```python
from build123d import *

# Parameters (mm, degrees)
SKETCH1_W                                  = 38
SKETCH1_H                                  = 38
BOSS_EXTRUDE1_DEPTH                        = 2
SKETCH2_R                                  = 2.25
BOSS_EXTRUDE2_DEPTH                        = 2
M3_TAPPED_HOLE1_D                          = 2.5
FILLET1_R                                  = 4
BOSS_EXTRUDE3_DEPTH                        = 1.5
SKETCH9_W                                  = 1.25
SKETCH9_H                                  = 1.5
SKETCH7_W                                  = 4.5
SKETCH7_H                                  = 2
BOSS_EXTRUDE4_DEPTH                        = 18
MIRROR1_AT_THE_SECOND_PLANE_COPY_1_SKETC_R = 2.25
MIRROR1_AT_THE_SECOND_PLANE_COPY_1_DEPTH   = 2
MIRROR1_AT_THE_SECOND_PLANE_COPY_2_D       = 2.5
MIRROR3_OUTLINE_W                          = 4.5
MIRROR3_OUTLINE_H                          = 2
MIRROR3_DEPTH                              = 19.5
MIRROR3_2_OUTLINE_R                        = 1.25
MIRROR3_2_DEPTH                            = 1.5


# Read off the part's stored shape, not the designer's step: Mirror3
with BuildPart() as part:
    # Sketch1 → Boss-Extrude1 (new body)
    with BuildSketch(Plane(origin=(0, 17.5, 0), x_dir=(1, 0, 0), z_dir=(0, 1, 0))):
        Rectangle(SKETCH1_W, SKETCH1_H)
    extrude(amount=BOSS_EXTRUDE1_DEPTH)

    # Sketch2 → Boss-Extrude2 (add)
    with BuildSketch(Plane(origin=(0, 19.5, 0), x_dir=(1, 0, 0), z_dir=(0, 1, 0))):
        with Locations(Location((15.25, 15.25, 0), (0, 0, 90))):
            Circle(SKETCH2_R)
    boss_extrude2 = extrude(amount=BOSS_EXTRUDE2_DEPTH)

    # M3 Tapped Hole1 (through all)
    with Locations(Plane(origin=(0, 21.5, 0), x_dir=(1, 0, 0), z_dir=(0, 1, 0))):
        with Locations((15.25, 15.25)):
            m3_tapped_hole1 = Hole(M3_TAPPED_HOLE1_D / 2)

    # Fillet1
    fillet1_edges = [part.edges().sort_by_distance(p)[0] for p in [
        (-19, 18.5, -19),
        (-19, 18.5, 19),
        (19, 18.5, 19),
        (19, 18.5, -19),
    ]]
    fillet(fillet1_edges, radius=FILLET1_R)



with BuildPart() as body_2:
    # Sketch6 → Boss-Extrude3 (new body)
    with BuildSketch(Plane(origin=(0, 0, 0), x_dir=(1, 0, 0), z_dir=(0, 1, 0))):
        with BuildLine():
            Line((13.25, 23), (13.25, 19))
            Line((13.25, 19), (8.75, 19))
            Line((8.75, 19), (8.75, 23))
            ThreePointArc((8.75, 23), (11, 25.25), (13.25, 23))
        make_face()
    extrude(amount=BOSS_EXTRUDE3_DEPTH)

    # Sketch9 → M3 Tapped Hole2 (revolve, cut)
    with BuildSketch(Plane(origin=(11, 1.5, -23), x_dir=(0, 0, 1), z_dir=(1, 0, 0))):
        with Locations((0.625, 0.75)):
            Rectangle(SKETCH9_W, SKETCH9_H)
    revolve(axis=Axis((11, 7.85, -23), (0, -1, 0)), mode=Mode.SUBTRACT)


with BuildPart() as part_1:
    add(part.part)

    add(body_2.part)  # Boss-Extrude4 merges body 2
    # Sketch7 → Boss-Extrude4 (add)
    with BuildSketch(Plane(origin=(0, 1.5, 0), x_dir=(1, 0, 0), z_dir=(0, 1, 0))):
        with Locations((11, 20)):
            Rectangle(SKETCH7_W, SKETCH7_H)
    extrude(amount=BOSS_EXTRUDE4_DEPTH)

    # Mirror1: Boss-Extrude2, M3 Tapped Hole1 across plane
    add(boss_extrude2.mirror(Plane(origin=(0, 0, 0), x_dir=(0, 0, 1), z_dir=(1, 0, 0))))
    add(m3_tapped_hole1.mirror(Plane(origin=(0, 0, 0), x_dir=(0, 0, 1), z_dir=(1, 0, 0))), mode=Mode.SUBTRACT)

    # Mirror1 at the second plane: Boss-Extrude2, M3 Tapped Hole1 across plane
    add(boss_extrude2.mirror(Plane.XY))
    add(m3_tapped_hole1.mirror(Plane.XY), mode=Mode.SUBTRACT)

    # Mirror1 at the second plane copy 1 sketc → Mirror1 at the second plane copy 1 (add)
    with BuildSketch(Plane(origin=(0, 19.5, 0), x_dir=(-1, 0, 0), z_dir=(0, 1, 0))):
        with Locations(Location((15.25, 15.25, 0), (0, 0, 90))):
            Circle(MIRROR1_AT_THE_SECOND_PLANE_COPY_1_SKETC_R)
    extrude(amount=MIRROR1_AT_THE_SECOND_PLANE_COPY_1_DEPTH)

    # Mirror1 at the second plane copy 2 (through all)
    with Locations(Plane(origin=(0, 21.5, 0), x_dir=(-1, 0, 0), z_dir=(0, 1, 0))):
        with Locations((15.25, 15.25)):
            Hole(MIRROR1_AT_THE_SECOND_PLANE_COPY_2_D / 2)

    # Mirror3 outline → Mirror3 (add)
    with BuildSketch(Plane(origin=(0, 0, 0), x_dir=(1, 0, 0), z_dir=(0, 1, 0))):
        with Locations((-11, -20)):
            Rectangle(MIRROR3_OUTLINE_W, MIRROR3_OUTLINE_H)
        with Locations((11, -20)):
            Rectangle(MIRROR3_OUTLINE_W, MIRROR3_OUTLINE_H)
        with Locations((-11, 20)):
            Rectangle(MIRROR3_OUTLINE_W, MIRROR3_OUTLINE_H)
    extrude(amount=MIRROR3_DEPTH)

    # Mirror3 2 outline → Mirror3 2 (add)
    # profile 1 of 3: a face of its own
    with BuildSketch(Plane(origin=(0, 0, 0), x_dir=(1, 0, 0), z_dir=(0, 1, 0))):
        with BuildLine():
            Line((13.25, -23), (13.25, -21))
            Line((13.25, -21), (8.75, -21))
            Line((8.75, -21), (8.75, -23))
            ThreePointArc((8.75, -23), (11, -25.25), (13.25, -23))
        make_face()
        with Locations((11, -23)):
            Circle(MIRROR3_2_OUTLINE_R, mode=Mode.SUBTRACT)
    # profile 2 of 3: a face of its own
    with BuildSketch(Plane(origin=(0, 0, 0), x_dir=(1, 0, 0), z_dir=(0, 1, 0))):
        with BuildLine():
            Line((-8.75, -23), (-8.75, -21))
            Line((-8.75, -21), (-13.25, -21))
            Line((-13.25, -21), (-13.25, -23))
            ThreePointArc((-13.25, -23), (-11, -25.25), (-8.75, -23))
        make_face()
        with Locations((-11, -23)):
            Circle(MIRROR3_2_OUTLINE_R, mode=Mode.SUBTRACT)
    # profile 3 of 3: a face of its own
    with BuildSketch(Plane(origin=(0, 0, 0), x_dir=(1, 0, 0), z_dir=(0, 1, 0))):
        with BuildLine():
            Line((-13.25, 21), (-8.75, 21))
            Line((-8.75, 21), (-8.75, 23))
            ThreePointArc((-8.75, 23), (-11, 25.25), (-13.25, 23))
            Line((-13.25, 23), (-13.25, 21))
        make_face()
        with Locations((-11, 23)):
            Circle(MIRROR3_2_OUTLINE_R, mode=Mode.SUBTRACT)
    extrude(amount=MIRROR3_2_DEPTH)


solid = part_1.part
```
Geometry: final body of the model. Coordinates: model frame, mm. A direction names the side the tool comes from. Round coordinates to 2 decimals unless told otherwise and drop trailing zeros. Order: outer loops, then holes, each group sorted by start corner. A loop starts at its lowest first (then second) coordinate and runs counter-clockwise, first axis right, second up. Notation, with made-up numbers: (-32, 49.5) -> (-22, 49.5) arc R7 ccw to (-22, 59.5) -> close; hole circle Ø5 at (45.5, 79). An arc over 180 degrees is marked (long way). Write each question's results on one line, items separated by ' | '.
Q1. Access query for faces 1 (the face through (-17.246, 20.486, 16.288)), 2 (the face through (-15, 21.5, -17)), 3 (the face through (14, 18, -19)), 4 (the face through (11, 9, -19)). Directions: +Z, -Z, +X, -X, +Y, -Y. A direction counts if a zero-diameter tool reaches every point of the face in a straight line with its end or side. Return the directions, or none.
Response values:
face 1: +Y | face 2: +Z, -Z, +X, -X, +Y | face 3: -Z, +X, +Y, -Y | face 4: +X, -X, -Y
Q2. Ray query, line 1 along Z through (x, y) = (11, 0.8); line 2 along Z through (x, y) = (12.5, 14.75); line 3 along Y through (x, z) = (17.5, -9). Return the intervals inside material, ascending.
Response values:
line 1: -25.25 to -24.25, -21.75 to -19, 19 to 21.75, 24.25 to 25.25 | line 2: -21 to -19, 19 to 21 | line 3: 17.5 to 19.5
Q3. Section query A-A (y = 8.75). Output: boundary loops of the cut face in (x, z).
Response values:
outline: (-13.25, -21) -> (-8.75, -21) -> (-8.75, -19) -> (-13.25, -19) -> close; (-13.25, 19) -> (-8.75, 19) -> (-8.75, 21) -> (-13.25, 21) -> close; (8.75, -21) -> (13.25, -21) -> (13.25, -19) -> (8.75, -19) -> close; (8.75, 19) -> (13.25, 19) -> (13.25, 21) -> (8.75, 21) -> close
Q4. Section query B-B (x = 11). Output: boundary loops of the cut face in (y, z), and give its area (3 significant figures).
Response values:
outline: (0, -25.25) -> (1.5, -25.25) -> (1.5, -24.25) -> (0, -24.25) -> close; (0, -21.75) -> (1.5, -21.75) -> (1.5, -21) -> (19.5, -21) -> (19.5, 21) -> (1.5, 21) -> (1.5, 21.75) -> (0, 21.75) -> (0, 19) -> (17.5, 19) -> (17.5, -19) -> (0, -19) -> close; (0, 24.25) -> (1.5, 24.25) -> (1.5, 25.25) -> (0, 25.25) -> close | area: 159 mm²
Q5. Section query C-C (z = 20). Output: boundary loops of the cut face in (x, y).
Response values:
outline: (-13.25, 0) -> (-8.75, 0) -> (-8.75, 19.5) -> (-13.25, 19.5) -> close; (8.75, 0) -> (13.25, 0) -> (13.25, 19.5) -> (8.75, 19.5) -> close
Q6. Pull-direction query (Z, two-part tool) for faces 5 (the face through (12, 1.5, 22)), 6 (the face through (11, 9, 19)), 7 (the face through (-11, 10, -21)); classes: released by +Z, released by -Z, zero draft, split by the parting line, or undercut.
Response values:
face 5: zero draft | face 6: undercut | face 7: released by -Z
Q7. Section query D-D (z = 2). Output: boundary loops of the cut face in (x, y).
Response values:
outline: (-19, 17.5) -> (19, 17.5) -> (19, 19.5) -> (-19, 19.5) -> close
Q8. Pin query (flat end, axial travel): pin 1 Ø1.3 at (x, z) = (-10, 22.5) entering from +Y; pin 2 Ø4.5 at (y, z) = (9, -20) entering from -X; pin 3 Ø0.9 at (x, y) = (-14, 19) entering from +Z. Return the tip coordinate at first contact, or that it passes through.
Response values:
pin 1: y = 1.5 | pin 2: x = -13.25 | pin 3: z = 19
